Autodesk Inventor part; units mm, degrees
ref_plane "Arbeitsebene1" through (-140, 120, 0) normal (0, 1, 0) x (1, 0, 0)
ref_plane "YZ Plane" through (0, 0, 0) normal (1, 0, 0) x (0, 1, 0)
ref_plane "XZ Plane" through (0, 0, 0) normal (0, 1, 0) x (-1, 0, 0)
sketch "Skizze3" plane through (0, 0, 0) normal (0, 0, 1) x (1, 0, 0)
  line L0 (0, 0) -> (-140, 0)
  line L1 (-140, 0) -> (-140, 120)
  line L2 (-140, 240) -> (0, 240)
  line L3 (0, 240) -> (0, 0)
  line L4 (-34.5565, 44.5) -> (-109.2584, 44.5) construction
  line L5 (-42.5521, 75.5) -> (-110.6291, 75.5) construction
  line L6 (-85.5, 104.3529) -> (-85.5, 36.2759) construction
  line L7 (-54.5, 102.2969) -> (-54.5, 32.1639) construction
  line L8 (-70, -15.9958) -> (-70, 12.0858) construction
  circle A0 centre (-70, 60) radius 11
  circle A1 centre (-85.5, 75.5) radius 1.5
  circle A2 centre (-85.5, 44.5) radius 1.5
  circle A3 centre (-54.5, 44.5) radius 1.5
  circle A4 centre (-54.5, 75.5) radius 1.5
  line L9 (-140, 120) -> (0, 120) construction
  line L10 (-140, 120) -> (-140, 240)
  line L11 (-139.4457, 80) -> (19.1397, 80) construction
  line L12 (12.4919, 138) -> (-57.0145, 138) construction
  line L13 (-25, 139.378) -> (-25, 104.3529) construction
  line L14 (-34.3, 147.3505) -> (-34.3, 112.3254) construction
  line L15 (-25, 102) -> (-34.3, 102) construction
  line L16 (-25, 105) -> (-34.3, 105)
  line L17 (-34.3, 99) -> (-25, 99)
  arc A5 (-25, 99) -> (-25, 105) centre (-25, 102) ccw
  arc A6 (-34.3, 105) -> (-34.3, 99) centre (-34.3, 102) ccw
  line L18 (-6.3901, 160) -> (-134.3919, 160) construction
  point P0 (-70, 0)
  point P1 (-70, 10)
  point P2 (-130, 80)
  point P3 (-137.8382, 80)
  point P4 (-130, 160)
  point P5 (-10, 160)
  point P6 (-10, 80)
  point P7 (-70, 230)
  point P8 (-34.3, 138)
  point P9 (-25, 138)
  point P10 (-29.65, 102)
  dimension "d4" = 240
  dimension "d5" = 140
  dimension "d6" = 31
  dimension "d7" = 31
  dimension "d8" = 15.5
  dimension "d9" = 15.5
  dimension "d10" = 60
  dimension "d11" = 22
  dimension "d12" = 3
  dimension "d13" = 3
  dimension "d14" = 3
  dimension "d15" = 3
  dimension "d22" = 10
  dimension "d23" = 10
  dimension "d24" = 10
  dimension "d25" = 10
  dimension "d26" = 10
  dimension "d34" = 10
  dimension "d35" = 9.3
  dimension "d36" = 18
  dimension "d37" = 25
  dimension "d38" = 3
  dimension "d43" = 36
  dimension "d44" = 80
  dimension "d45" = 80
extrude "Extrusion3" add sketch "Skizze3" against normal blind 5 contours L0 L1 L10 L2 L3 | A0 | A1 | A2 | A3 | A4 | A5 L17 A6 L16
fillet "Rundung1" radius 2 4 edges at (0, 0, -2.5) (0, 240, -2.5) (-140, 240, -2.5) (-140, 0, -2.5)
ref_plane "Arbeitsebene1" through (-140, 120, 0) normal (0, 1, 0) x (1, 0, 0)
extrude "Extrusion4" cut sketch "Skizze3" against normal through all contours A0 | A1 | A2 | A3 | A4
mirror "Spiegeln1" about plane through (-140, 120, 0) normal (0, 1, 0) of "Extrusion4"
hole "Bohrung1" at (-70, 60, 0) at (-70, 10, 0) at (-130, 80, 0) at (-130, 160, 0) at (-10, 160, 0) at (-10, 80, 0) at (-70, 230, 0) direction (0, 0, -1) diameter 5.5 end through all
extrude "Extrusion5" cut sketch "Skizze3" against normal blind 10 contours A5 L17 A6 L16
hole "Bohrung2" at (-25, 138, 0) at (-34.3, 138, 0) direction (0, 0, -1) diameter 1.567 depth 4 tip angle 118
equation "\"d36\" = 0.5 * d43"
properties part number "BT001_trajan20_21" material "Acryl"
Model file for the job. Use its own axes, mm. A direction names the side the tool comes from. Round coordinates to 2 decimals unless told otherwise and drop trailing zeros. Write each loop counter-clockwise with the first axis right and the second up, starting at its lowest first coordinate (ties: lowest second). Pieces come first, ordered by that corner, then holes. Notation, with made-up numbers: (66, -6) -> (98, -6) arc R18 cw to (98, -1) -> close; hole circle Ø3 at (25, -28.75). An arc over 180 degrees is marked (long way). Answer as CSV lines item,"result".
1. Slice it at B-B, the plane y = 160. List the corners of the cut face in (x, z), plus the area to 3 significant figures.
Resolved:
outline,"(-140, -5) -> (-132.75, -5) -> (-132.75, 0) -> (-140, 0) -> close; (-127.25, -5) -> (-12.75, -5) -> (-12.75, 0) -> (-127.25, 0) -> close; (-7.25, -5) -> (0, -5) -> (0, 0) -> (-7.25, 0) -> close"
area,"645 mm²"
2. Slice it at D-D, the plane y = 56. List the corners of the cut face in (x, z).
Resolved:
outline,"(-140, -5) -> (-80.25, -5) -> (-80.25, 0) -> (-140, 0) -> close; (-59.75, -5) -> (0, -5) -> (0, 0) -> (-59.75, 0) -> close"
3. Slice it at A-A, the plane x = -70. List the corners of the cut face in (y, z).
Resolved:
outline,"(0, -5) -> (7.25, -5) -> (7.25, 0) -> (0, 0) -> close; (12.75, -5) -> (49, -5) -> (49, 0) -> (12.75, 0) -> close; (71, -5) -> (169, -5) -> (169, 0) -> (71, 0) -> close; (191, -5) -> (227.25, -5) -> (227.25, 0) -> (191, 0) -> close; (232.75, -5) -> (240, -5) -> (240, 0) -> (232.75, 0) -> close"
4. Pin check, flat tip, straight feed: pin 1 Ø2.5 at (x, y) = (-54.5, 195.5) entering from +Z. Stop position of the tip, or through.
Resolved:
pin 1,"through"
5. Drill centre lines: line 1 (X direction, y = 160, z = -1.3); line 2 (Y direction, x = -54.5, z = -3.45); line 3 (X direction, y = 138, z = -2.95). Where is each one in solid material? Low to high.
Resolved:
line 1,"-140 to -132.75, -127.25 to -12.75, -7.25 to 0"
line 2,"0 to 43, 46 to 74, 77 to 163, 166 to 194, 197 to 240"
line 3,"-140 to -35.08, -33.52 to -25.78, -24.22 to 0"
6. Slice it at C-C, the plane y = 230. List the corners of the cut face in (x, z).
Resolved:
outline,"(-140, -5) -> (-72.75, -5) -> (-72.75, 0) -> (-140, 0) -> close; (-67.25, -5) -> (0, -5) -> (0, 0) -> (-67.25, 0) -> close"
7. Tool access for faces 4 (the face through (-30, 99, -2)), 5 (the face through (-140, 118, -2)): list every direction of +Z, -Z, +X, -X, +Y, -Y with a clear straight run to the whole face (end or side of a thin tool).
Resolved:
face 4,"+Z, -Z"
face 5,"+Z, -Z, -X, +Y, -Y"
8. Mould opens along Y. For faces 1 (the face through (-69, 0, -2)), 2 (the face through (-71, 122, 0)), 3 (the face through (-127.315, 80.596, -2.535)) say: +Y half, -Y half, draft (parallel to the pull), parting line (faces both ways), or undercut.
Resolved:
face 1,"-Y half"
face 2,"draft"
face 3,"undercut"
